Here's how the part is built. I have some questions about the finished solid (model axes, mm). A direction names the side the tool comes from. Coordinates: 2 decimals unless noted, no trailing zeros. Loops run counter-clockwise (first coordinate to the right, second up) from the corner with the lowest first, then second, coordinate; pieces in that order, holes last.
from build123d import *

# Parameters (mm, degrees)
F0_W     = 203.2
F0_H     = 203.2
F0_W_2   = 19.05
F0_W_3   = 12.7
F0_W_4   = 260.35
F1_DEPTH = 19.05
F2_DEPTH = 6.35


with BuildPart() as f1:
    # F0 (on Right) → F1 (new body)
    with BuildSketch(Plane.YZ):
        with Locations((152.4, 0)):
            Rectangle(F0_W, F0_H)
        with Locations((28.575, 0)):
            Rectangle(F0_W_2, F0_H)
        with Locations((12.7, 0)):
            Rectangle(F0_W_3, F0_H)
        with Locations((-123.825, 0)):
            Rectangle(F0_W_4, F0_H)
        with Locations((44.45, 0)):
            Rectangle(F0_W_3, F0_H)
    extrude(amount=-F1_DEPTH)

    # F0 (on Right) → F2 (join)
    with BuildSketch(Plane.YZ):
        with Locations((44.45, 0)):
            Rectangle(F0_W_3, F0_H)
        with Locations((12.7, 0)):
            Rectangle(F0_W_3, F0_H)
    extrude(amount=F2_DEPTH)


solid = f1.part
Q1. Will these pins go through, and if not, where does the flat tip stop? P1, Ø1.9, axis at x = 4, z = -45, coming from the +Y side; P2, Ø3, axis at y = -75, z = -41, coming from the +X side; P3, Ø2, axis at x = 2, y = -81.5, coming from the -Z side; P4, Ø5, axis at x = 3.5, z = -1.5, coming from the -Y side.
Q2. For faces 1 (the flat face through (-9, 4, 101.6)), 2 (the flat face through (0, 151, 1)), 3 (the flat face through (0, -126, 1)), which set-ups out of +Z, -Z, +X, -X, +Y, -Y let a thin tool reach every point of the face, with its end or its side?
Q3. Please list where this line runs through material, in increasing order: probe 1 along X at (y, z) = (76.5, 5).
Q4. We'd pull the mould along Y, two halves only. Please class faces 4 (the flat face through (-9, -254, -1)), 5 (the flat face through (0, 28, 1)), 6 (the flat face through (-9, 254, -1)), 7 (the flat face through (6.35, 13, 1)): pulls with the +Y half, pulls with the -Y half, needs draft (parallel to the pull), parting line crosses it, or undercut.
Q5. Suppose I cut it at A-A on z = -25. Write out the boundary of the cut face in (x, y).
Q6. Suppose I cut it at B-B on y = -12.5. Write out the boundary of the cut face in (x, z), and give its area (3 significant figures).
Check values:
1. P1: stops at y = 50.8
1. P2: stops at x = 0
1. P3: passes through
1. P4: stops at y = 6.35
2. face 1: +Z, +X, -X, +Y, -Y
2. face 2: +Z, -Z, +X, +Y
2. face 3: +Z, -Z, +X, -Y
3. probe 1: x = -19.05 to 0
4. face 4: pulls with the -Y half
4. face 5: undercut
4. face 6: pulls with the +Y half
4. face 7: needs draft
5. outline: (-19.05, -254) - (0, -254) - (0, 6.35) - (6.35, 6.35) - (6.35, 19.05) - (0, 19.05) - (0, 38.1) - (6.35, 38.1) - (6.35, 50.8) - (0, 50.8) - (0, 254) - (-19.05, 254) - close
6. outline: (-19.05, -101.6) - (0, -101.6) - (0, 101.6) - (-19.05, 101.6) - close
6. area: 3,870 mm2
